Check sheet for the modelled part. Datum: model origin and axes. Units: mm. A direction names the side the tool comes from. Coordinates: 2 decimals unless noted, no trailing zeros. Loops run counter-clockwise (first coordinate to the right, second up) from the corner with the lowest first, then second, coordinate; pieces in that order, holes last. Notation, with made-up numbers: (-16.5, -30) - (13.5, -30) arc R30 ccw to (13.5, -8) - close; hole circle Ø4 at (11.25, 63). An arc over 180 degrees is marked (long way). Use a Markdown table: item, result. Add a question column.
1) Tool access check on faces 1 (the cylindrical face through (-0.29, 2.73, -2.23)), 2 (the cylindrical face through (-2.17, 0.99, 9.76)). Record the directions out of +Z, -Z, +X, -X, +Y, -Y that give a thin tool (end or side, any length) a straight path to the whole face; none if there is none.
2) Draft check along Z on faces 3 (the flat face through (0, 0, 2)), 4 (the cylindrical face through (-1.5, 0.44, -0.07)), 5 (the cylindrical face through (-0.59, 3.23, -4.46)). Enter one of: pulls with the +Z half, pulls with the -Z half, needs draft (parallel to the pull), parting line crosses it, or undercut.
3) Sectioned sample at D-D, the plane y = 3.55. Enter the section's corners in (x, z).
4) Go/stop test with flat-tipped pins: P1, Ø4, axis at x = 4.95, z = -4.95, coming from the +Y side; P2, Ø3, axis at x = -3, z = 4.5, coming from the +Y side; P3, Ø4, axis at x = 0, z = 0, coming from the +Y side; P4, Ø2, axis at x = -4, y = 2, coming from the -Z side. Record where each tip stops, or that it passes through.
5) Sectioned sample at B-B, the plane x = 0. Enter the section's corners in (y, z), then the cut area to 3 significant figures.
6) Sectioned sample at C-C, the plane z = 4. Enter the section's corners in (x, y).
7) Thickness scan on line 1 (X direction, y = 0.6, z = 0); line 2 (X direction, y = 1.85, z = -6); line 3 (X direction, y = 1, z = -5.5). Record the ranges inside material, lowest first.
8) Sectioned sample at A-A, the plane z = 0. Enter the section's corners in (x, y), then the cut area to 3 significant figures.
from build123d import *

# Parameters (mm, degrees)
SKETCH1_R           = 10
SKETCH1_R_2         = 1.25
SKETCH1_R_3         = 1.5
BOSS_EXTRUDE1_DEPTH = 2
SKETCH2_R           = 4.5
SKETCH2_R_2         = 1.5
BOSS_EXTRUDE2_DEPTH = 2.5
SKETCH3_R           = 2.25
CUT_EXTRUDE1_DEPTH  = 3.6


with BuildPart() as part:
    # Sketch1 → Boss-Extrude1 (new body)
    with BuildSketch(Plane(origin=(0, 0, 0), x_dir=(1, 0, 0), z_dir=(0, 1, 0))):
        Circle(SKETCH1_R)
        with Locations((-4.949747468, 4.949747468)):
            Circle(SKETCH1_R_2, mode=Mode.SUBTRACT)
        with Locations((4.949747468, 4.949747468)):
            Circle(SKETCH1_R_2, mode=Mode.SUBTRACT)
        with Locations((4.949747468, -4.949747468)):
            Circle(SKETCH1_R_2, mode=Mode.SUBTRACT)
        with Locations((-4.949747468, -4.949747468)):
            Circle(SKETCH1_R_2, mode=Mode.SUBTRACT)
        Circle(SKETCH1_R_3, mode=Mode.SUBTRACT)
    extrude(amount=BOSS_EXTRUDE1_DEPTH)

    # Sketch2 → Boss-Extrude2 (add)
    with BuildSketch(Plane(origin=(0, 2, 0), x_dir=(1, 0, 0), z_dir=(0, 1, 0))):
        Circle(SKETCH2_R)
        Circle(SKETCH2_R_2, mode=Mode.SUBTRACT)
    extrude(amount=BOSS_EXTRUDE2_DEPTH)

    # Sketch3 → Cut-Extrude1 (cut)
    with BuildSketch(Plane(origin=(0, 4.5, 0), x_dir=(1, 0, 0), z_dir=(0, 1, 0))):
        Circle(SKETCH3_R)
    extrude(amount=-CUT_EXTRUDE1_DEPTH, mode=Mode.SUBTRACT)


solid = part.part
Solved:
| question | item | result |
|---|---|---|
| 1 | face 1 | +Y |
| 1 | face 2 | +Y, -Y |
| 2 | face 3 | needs draft |
| 2 | face 4 | undercut |
| 2 | face 5 | parting line crosses it |
| 3 | outline | circle Ø9 at (0, 0); hole circle Ø4.5 at (0, 0) |
| 4 | P1 | stops at y = 2 |
| 4 | P2 | stops at y = 4.5 |
| 4 | P3 | stops at y = 0.9 |
| 4 | P4 | stops at z = -9.54 |
| 5 | outline | (0, -10) - (2, -10) - (2, -4.5) - (4.5, -4.5) - (4.5, -2.25) - (0.9, -2.25) - (0.9, -1.5) - (0, -1.5) - close; (0, 1.5) - (0.9, 1.5) - (0.9, 2.25) - (4.5, 2.25) - (4.5, 4.5) - (2, 4.5) - (2, 10) - (0, 10) - close |
| 5 | area | 43.6 mm2 |
| 6 | outline | (-9.17, 0) - (-5.76, 0) - (-5.76, 2) - (-9.17, 2) - close; (-4.14, 0) - (4.14, 0) - (4.14, 2) - (2.06, 2) - (2.06, 4.5) - (-2.06, 4.5) - (-2.06, 2) - (-4.14, 2) - close; (5.76, 0) - (9.17, 0) - (9.17, 2) - (5.76, 2) - close |
| 7 | line 1 | x = -10 to -1.5, 1.5 to 10 |
| 7 | line 2 | x = -8 to -5.63, -4.27 to 4.27, 5.63 to 8 |
| 7 | line 3 | x = -8.35 to -6.07, -3.83 to 3.83, 6.07 to 8.35 |
| 8 | outline | (-10, 0) - (-1.5, 0) - (-1.5, 0.9) - (-2.25, 0.9) - (-2.25, 4.5) - (-4.5, 4.5) - (-4.5, 2) - (-10, 2) - close; (1.5, 0) - (10, 0) - (10, 2) - (4.5, 2) - (4.5, 4.5) - (2.25, 4.5) - (2.25, 0.9) - (1.5, 0.9) - close |
| 8 | area | 43.6 mm2 |
